```python
from build123d import *

# Parameters (mm, degrees)
SKETCH1_R           = 2.75
BOSS_EXTRUDE1_DEPTH = 3
SKETCH5_R           = 5.226301297
SKETCH5_R_2         = 1.5
CUT_EXTRUDE2_DEPTH  = 7.2


with BuildPart() as part:
    # Sketch1 → Boss-Extrude1 (new body)
    with BuildSketch(Plane(origin=(0, 0, 0), x_dir=(1, 0, 0), z_dir=(0, 1, 0))):
        with BuildLine():
            Line((-4.5, 31.251652173), (-4.5, 12.196310918))
            ThreePointArc((-4.5, 12.196310918), (-9.192388155, 9.192388155), (-12.196310918, 4.5))
            Line((-12.196310918, 4.5), (-31.251652173, 4.5))
            ThreePointArc((-31.251652173, 4.5), (-38.523072163, 0), (-31.251652173, -4.5))
            Line((-31.251652173, -4.5), (-12.196310918, -4.5))
            ThreePointArc((-12.196310918, -4.5), (-9.192388155, -9.192388155), (-4.5, -12.196310918))
            Line((-4.5, -12.196310918), (-4.5, -31.251652173))
            ThreePointArc((-4.5, -31.251652173), (0, -38.523072163), (4.5, -31.251652173))
            Line((4.5, -31.251652173), (4.5, -12.196310918))
            ThreePointArc((4.5, -12.196310918), (9.192388155, -9.192388155), (12.196310918, -4.5))
            Line((12.196310918, -4.5), (31.251652173, -4.5))
            ThreePointArc((31.251652173, -4.5), (38.523072163, 0), (31.251652173, 4.5))
            Line((31.251652173, 4.5), (12.196310918, 4.5))
            ThreePointArc((12.196310918, 4.5), (9.192388155, 9.192388155), (4.5, 12.196310918))
            Line((4.5, 12.196310918), (4.5, 31.251652173))
            ThreePointArc((4.5, 31.251652173), (0, 38.523072163), (-4.5, 31.251652173))
        make_face()
        with Locations(Location((0, -33.494924376, 0), (0, 0, 270))):
            Circle(SKETCH1_R, mode=Mode.SUBTRACT)
        with Locations(Location((-33.494924376, 0, 0), (0, 0, 270))):
            Circle(SKETCH1_R, mode=Mode.SUBTRACT)
        with Locations(Location((0, 33.494924376, 0), (0, 0, 270))):
            Circle(SKETCH1_R, mode=Mode.SUBTRACT)
        with Locations(Location((33.494924376, 0, 0), (0, 0, 270))):
            Circle(SKETCH1_R, mode=Mode.SUBTRACT)
    extrude(amount=BOSS_EXTRUDE1_DEPTH)

    # Chamfer1
    # the kernel refuses this chamfer: 5 mm, written as the material it adds along each edge
    with BuildSketch(Plane(origin=(-12.196310918, 0, -4.5), x_dir=(0.4944512114841002, 0, -0.869205383935181), z_dir=(0, 1, 0)), Plane(origin=(4.5, 0, -12.196310918), x_dir=(0.8692053839351812, 0, 0.4944512114841002), z_dir=(0, 1, 0)), Plane(origin=(12.196310918, 0, 4.5), x_dir=(-0.4944512114841005, 0, 0.869205383935181), z_dir=(0, 1, 0)), Plane(origin=(-4.5, 0, 12.196310918), x_dir=(-0.869205383935182, 0, -0.4944512114840988), z_dir=(0, 1, 0))) as chamfer1_piece_1:
        with BuildLine():
            Line((3.583193205, 0), (-2.272552352, 3.809310984))
            Line((-2.272552352, 3.809310984), (-2.359472891, 3.759865863))
            ThreePointArc((-2.359472891, 3.759865863), (-1.183301792, 1.877904769), (-0.086920538, -0.049445121))
            Line((-0.086920538, -0.049445121), (0.016300434, -0.098662535))
            ThreePointArc((0.016300434, -0.098662535), (1.789817923, 0.069668276), (3.573220218, -0.099501455))
            Line((3.573220218, -0.099501455), (3.583193205, 0))
        make_face()
    extrude(amount=3)
    with BuildSketch(Plane(origin=(-4.5, 0, -12.196310918), x_dir=(0.020694934032123476, 0, -0.9997858369197905), z_dir=(0, 1, 0)), Plane(origin=(12.196310918, 0, -4.5), x_dir=(0.9997858369197905, 0, 0.020694934032131303), z_dir=(0, 1, 0)), Plane(origin=(4.5, 0, 12.196310918), x_dir=(-0.020694934032078793, 0, 0.9997858369197915), z_dir=(0, 1, 0)), Plane(origin=(-12.196310918, 0, 4.5), x_dir=(-0.9997858369197906, 0, -0.020694934032118258), z_dir=(0, 1, 0))) as chamfer1_piece_2:
        with BuildLine():
            Line((4.435689841, 0), (-1.835789795, 3.077198299))
            Line((-1.835789795, 3.077198299), (-1.916130816, 3.017655706))
            ThreePointArc((-1.916130816, 3.017655706), (-0.857153439, 1.572765033), (-0.093081321, -0.036549524))
            Line((-0.093081321, -0.036549524), (0.002069493, -0.099978584))
            ThreePointArc((0.002069493, -0.099978584), (2.218964555, -0.054090259), (4.437759335, -0.099978584))
            Line((4.437759335, -0.099978584), (4.435689841, 0))
        make_face()
    extrude(amount=3)

    # Sketch5 → Cut-Extrude2 (cut)
    with BuildSketch(Plane(origin=(0, 3, 0), x_dir=(1, 0, 0), z_dir=(0, 1, 0))):
        with Locations(Location((0, 0, 0), (0, 0, 270))):
            Circle(SKETCH5_R)
        with Locations(Location((-1.03e-07, 12, 0), (0, 0, 270))):
            Circle(SKETCH5_R_2)
        with Locations(Location((12, 1.03e-07, 0), (0, 0, 270))):
            Circle(SKETCH5_R_2)
        with Locations(Location((1.03e-07, -12, 0), (0, 0, 270))):
            Circle(SKETCH5_R_2)
        with Locations(Location((-12, -1.03e-07, 0), (0, 0, 270))):
            Circle(SKETCH5_R_2)
    extrude(amount=-CUT_EXTRUDE2_DEPTH, mode=Mode.SUBTRACT)


solid = part.part
```
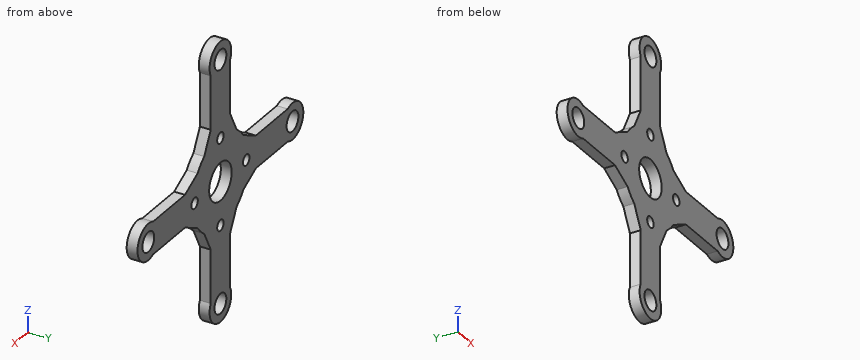
The model under review builds one solid part; all positions refer to its coordinate system, in mm. Round coordinates to 2 decimals unless told otherwise and drop trailing zeros. Loops run counter-clockwise (first coordinate to the right, second up) from the corner with the lowest first, then second, coordinate; pieces in that order, holes last. Notation, with made-up numbers: M 50,71.25 L 58,71.25 A28 ccw 58,105.25 Z; hole C -30,7 d10. An arc over 180 degrees is marked long. Write item = value, one per line.
Item 1: Insertion check: P1, Ø5, axis at x = 12, z = 0, coming from the -Y side; P2, Ø0.9, axis at x = 21, y = 2, coming from the -Z side; P3, Ø0.9, axis at x = 25.5, y = 1.5, coming from the +Z side; P4, Ø2.5, axis at x = 0, z = 12, coming from the -Y side. Each pin has a flat end and moves straight along its axis. Give the tip position at first contact, or say it passes through.
Return value:
P1 = 0
P2 = -4.5
P3 = 4.5
P4 = through
Item 2: Take a section at D-D on y = 1.8. State how many separate pieces and enclosed holes the cut face has, then the cut area to 3 significant figures.
Return value:
separate_pieces = 1
enclosed_holes = 9
area = 1,280 mm2
Item 3: Take a section at B-B on z = 0. Write out the cut boundary in (x, y), then the cut area to 3 significant figures.
Return value:
outline = M -38.52,0 L -36.24,0 L -36.24,3 L -38.52,3 Z; M -30.74,0 L -13.5,0 L -13.5,3 L -30.74,3 Z; M -10.5,0 L -5.23,0 L -5.23,3 L -10.5,3 Z; M 5.23,0 L 10.5,0 L 10.5,3 L 5.23,3 Z; M 13.5,0 L 30.74,0 L 30.74,3 L 13.5,3 Z; M 36.24,0 L 38.52,0 L 38.52,3 L 36.24,3 Z
area = 149 mm2
Item 4: Take a section at A-A on x = 0. Write out the cut boundary in (y, z), then the cut area to 3 significant figures.
Return value:
outline = M 0,-38.52 L 3,-38.52 L 3,-36.24 L 0,-36.24 Z; M 0,-30.74 L 3,-30.74 L 3,-13.5 L 0,-13.5 Z; M 0,-10.5 L 3,-10.5 L 3,-5.23 L 0,-5.23 Z; M 0,5.23 L 3,5.23 L 3,10.5 L 0,10.5 Z; M 0,13.5 L 3,13.5 L 3,30.74 L 0,30.74 Z; M 0,36.24 L 3,36.24 L 3,38.52 L 0,38.52 Z
area = 149 mm2
Item 5: For line 1 (Z direction, x = -2.5, y = 0.7); line 2 (Z direction, x = -0.5, y = 1.3); line 3 (Z direction, x = -25, y = 1.4), list the stretches that pass through material, from the lowest coordinate up. Write a range as [from, to].
Return value:
line_1 = [-37.86, -34.64], [-32.35, -4.59], [4.59, 32.35], [34.64, 37.86]
line_2 = [-38.5, -36.2], [-30.79, -13.41], [-10.59, -5.2], [5.2, 10.59], [13.41, 30.79], [36.2, 38.5]
line_3 = [-4.5, 4.5]
Item 6: Take a section at C-C on z = 12. Write out the cut boundary in (x, y).
Return value:
outline = M -6.8,0 L -1.5,0 L -1.5,3 L -6.8,3 Z; M 1.5,0 L 6.8,0 L 6.8,3 L 1.5,3 Z
